Input: part model. Units: mm. Frame: model coordinates. A direction names the side the tool comes from. Give positions to 0.01 mm unless a question says otherwise; leave off trailing zeros. Write each loop counter-clockwise with the first axis right and the second up, starting at its lowest first coordinate (ties: lowest second). Pieces come first, ordered by that corner, then holes. Notation, with made-up numbers: (-36, -9.5) - (21, -9.5) arc R8 ccw to (21, 1.5) - close; hole circle Ø4 at (79, 64). An arc over 180 degrees is marked (long way). Answer as a JSON object with one key per item and string values. Group by question number.
from build123d import *

# Parameters (mm, degrees)
SKETCH005_W   = 10.037777
SKETCH005_H   = 4.545547
PAD003_DEPTH  = 23
SKETCH004_W   = 36.161861
SKETCH004_H   = 4.748486
PAD002_DEPTH  = 100
PAD001_DEPTH  = 50
ARRAY_Y_COUNT = 7
ARRAY_Y_PITCH = 10
SKETCH_R      = 1.75
PAD_DEPTH     = 9
FILLET_R      = 1
FILLET002_R   = 3


with BuildPart() as pad003:
    # Sketch005 → Pad003 (new body, symmetric)
    with BuildSketch(Plane.YZ.offset(1)):
        with Locations((-0.053055, 6.772661)):
            Rectangle(SKETCH005_W, SKETCH005_H)
    extrude(amount=PAD003_DEPTH, both=True)


with BuildPart() as pad002:
    # Sketch004 → Pad002 (new body)
    with BuildSketch(Plane(origin=(1, -50, 0), x_dir=(1, 0, 0), z_dir=(0, -1, 0))):
        with Locations((0.005565, 6.850441)):
            Rectangle(SKETCH004_W, SKETCH004_H)
    extrude(amount=-PAD002_DEPTH)


with BuildPart() as array:
    # Sketch003 → Pad001 (new body)
    with BuildSketch(Plane(origin=(-23.0697, 0, 0), x_dir=(0, -1, 0), z_dir=(-1, 0, 0))):
        with BuildLine():
            Line((-1.127729, 2.982091), (2.228669, 6.982091))
            ThreePointArc((3.377736, 6.017909), (3.285293, 7.074533), (2.228669, 6.982091))
            Line((0.021337, 2.017909), (3.377736, 6.017909))
            ThreePointArc((-1.127729, 2.982091), (-1.035287, 1.925467), (0.021337, 2.017909))
        make_face()
    extrude(amount=-PAD001_DEPTH)

    # Array Y: Array ×7


with BuildPart() as array_1:
    add(array.part)
    with Locations(*[(0, i * ARRAY_Y_PITCH, 0) for i in range(1, ARRAY_Y_COUNT)]):
        add(array.part)


with BuildPart() as array_2:
    # Array placement: moved
    add(array_1.part.moved(Location((0, -29.5, 0))))


with BuildPart() as cut002:
    # Sketch → Pad (new body)
    with BuildSketch(Plane.XY):
        Polygon((-12.0697, 41.4218), (13.9303, 41.4218), (24.322605, 47.4218), (29.822605, 37.895521), (24.9303, 35.070947), (24.9303, -36.227347), (29.822605, -39.051921), (24.322605, -48.5782), (13.9303, -42.5782), (-12.0697, -42.5782), (-22.462005, -48.5782), (-27.962005, -39.051921), (-23.0697, -36.227347), (-23.0697, 35.070947), (-27.962005, 37.895521), (-22.462005, 47.4218), align=None)
        with Locations((-20.37566, -40.791855)):
            Circle(SKETCH_R, mode=Mode.SUBTRACT)
        with Locations((22.23626, -40.791855)):
            Circle(SKETCH_R, mode=Mode.SUBTRACT)
        with Locations((22.23626, 39.635455)):
            Circle(SKETCH_R, mode=Mode.SUBTRACT)
        with Locations((-20.37566, 39.635455)):
            Circle(SKETCH_R, mode=Mode.SUBTRACT)
        Polygon((22.9303, 35.070947), (22.9303, -36.227347), (17.35405, -40.5782), (-15.49345, -40.5782), (-21.0697, -36.227347), (-21.0697, 35.070947), (-15.49345, 39.4218), (17.35405, 39.4218), align=None, mode=Mode.SUBTRACT)
    extrude(amount=PAD_DEPTH)

    # Fillet
    fillet_edges = [cut002.edges().sort_by_distance(p)[0] for p in [
        (-22.462005, 47.4218, 4.5),
        (24.322605, 47.4218, 4.5),
        (29.822605, 37.895521, 4.5),
        (29.822605, -39.051921, 4.5),
        (24.322605, -48.5782, 4.5),
        (-22.462005, -48.5782, 4.5),
        (-27.962005, -39.051921, 4.5),
        (-27.962005, 37.895521, 4.5),
    ]]
    fillet(fillet_edges, radius=FILLET_R)

    # Cut: cut Array
    add(array_2.part, mode=Mode.SUBTRACT)

    # Cut001: cut Pad002
    add(pad002.part, mode=Mode.SUBTRACT)

    # Fillet002
    fillet002_edges = [cut002.edges().sort_by_distance(p)[0] for p in [
        (-17.075366, -39.343915, 6.738099),
        (-17.075366, -45.468223, 6.738099),
        (19.086495, -45.555131, 6.738099),
        (19.086495, -39.226465, 6.738099),
        (-17.075366, 44.311823, 6.738099),
        (-17.075366, 38.187515, 6.738099),
        (19.086495, 44.398731, 6.738099),
        (19.086495, 38.070065, 6.738099),
    ]]
    fillet(fillet002_edges, radius=FILLET002_R)

    # Cut002: cut Pad003
    add(pad003.part, mode=Mode.SUBTRACT)


solid = cut002.part
1) Mould query, pull axis Y, two halves, no side actions, for faces 6 (the face through (-22.084, 19.973, 4.954)), 7 (the face through (-22.084, -11.176, 3.99)), 8 (the face through (27.041, 42.713, 4.437)), 9 (the face through (-17.49, -45.26, 6.77)). Classes: +Y half, -Y half, draft (parallel to the pull), parting line (faces both ways), or undercut.
2) Line query: line 1 along X through (y, z) = (-26.5, 6.75); line 2 along Y through (x, z) = (5.5, 0.5); line 3 along X through (y, z) = (-4, 4.75). Output: solid intervals per line, ascending. Write a range as from..to.
3) Cut plane B-B on y = -14. Return the cut outline in (x, z), and give its area (3 significant figures).
4) Pin query (flat end, axial travel): P1, Ø2, axis at y = -16, z = 4.5, coming from the -X side; P2, Ø5, axis at x = -0.5, z = 2, coming from the -Y side; P3, Ø0.5, axis at x = 23.5, y = -3, coming from the +Z side. Return the tip coordinate at first contact, or that it passes through.
5) Reachability of faces 1 (the face through (-22.084, -30.027, 4.954)), 2 (the face through (26.915, -37.373, 4.437)), 3 (the face through (20.723, 36.793, 3.437)), 4 (the face through (19.5, 44.19, 6.71)), 5 (the face through (-23.07, -1, 3)) from +Z, -Z, +X, -X, +Y, -Y: full face, straight path, thin tool, end or side. Return the list, or none.
6) Cut plane A-A on x = 6. Return the cut outline in (y, z), and give its area (3 significant figures).
Filled in:
{
 "1": {"face 6": "undercut", "face 7": "undercut", "face 8": "+Y half", "face 9": "-Y half"},
 "2": {"line 1": "x = -23.07..-21.07, 22.93..24.93", "line 2": "y = -42.58..-40.58, 39.42..41.42", "line 3": "x = -23.07..-22, 24..24.93"},
 "3": {"outline": "(-23.07, 0) - (-21.07, 0) - (-21.07, 9) - (-23.07, 9) - close; (22.93, 0) - (24.93, 0) - (24.93, 9) - (22.93, 9) - close", "area": "36.0 mm²"},
 "4": {"P1": "stops at x = -23.07", "P2": "stops at y = -42.58", "P3": "stops at z = 4.5"},
 "5": {"face 1": "+X, -X", "face 2": "+Z, -Z, +X", "face 3": "+Z, -Z", "face 4": "+Z, +Y", "face 5": "+Z, -Z, -X"},
 "6": {"outline": "(-42.58, 0) - (-40.58, 0) - (-40.58, 4.48) - (-42.58, 4.48) - close; (39.42, 0) - (41.42, 0) - (41.42, 4.48) - (39.42, 4.48) - close", "area": "17.9 mm²"}
}
